Here's how the part is built. I have some questions about the finished solid (model axes, mm). A direction names the side the tool comes from. Give positions to 0.01 mm unless a question says otherwise; leave off trailing zeros. Write each loop counter-clockwise with the first axis right and the second up, starting at its lowest first coordinate (ties: lowest second). Pieces come first, ordered by that corner, then holes. Notation, with made-up numbers: (43, 65.5) - (63, 65.5) arc R32 ccw to (63, 100.5) - close; hole circle Ø2 at (11, 63). An arc over 180 degrees is marked (long way). Use a Markdown table: item, result.
```python
from build123d import *

# Parameters (mm, degrees)
POCKET_DEPTH = 0.75


with BuildPart() as part:
    # Sketch → Revolution (revolve)
    with BuildSketch(Plane.XZ):
        with BuildLine():
            Line((0, 0), (0, 11.75))
            Line((0, 11.75), (2.25, 11.75))
            ThreePointArc((3, 11), (2.78033, 11.53033), (2.25, 11.75))
            Line((3, 11), (3, 10))
            Line((3, 10), (1.5, 10))
            Line((1.5, 10), (1.5, 0))
            Line((1.5, 0), (0, 0))
        make_face()
    revolve(axis=Axis((0, 0, 0), (0, 0, 1)))

    # Sketch001 (on Face5 of Revolution) → Pocket (cut)
    with BuildSketch(Plane(origin=(0, 0, 11.75), x_dir=(-1, 0, 0), z_dir=(0, 0, 1))):
        Polygon((-3.274783, -2.372712), (2.184691, 3.4031), (3.274783, 2.372712), (-2.184691, -3.4031), align=None)
    extrude(amount=-POCKET_DEPTH, mode=Mode.SUBTRACT)


solid = part.part
```
Item 1: If we section it at C-C, the plane z = 8.5: Write out the boundary of the cut face in (x, y).
Values:
| item | result |
|---|---|
| outline | circle Ø3 at (0, 0) |
Item 2: If we section it at B-B, the plane x = 0: Write out the boundary of the cut face in (y, z), plus the area to 3 significant figures.
Values:
| item | result |
|---|---|
| outline | (-3, 10) - (-1.5, 10) - (-1.5, 0) - (1.5, 0) - (1.5, 10) - (3, 10) - (3, 11) arc R0.75 ccw to (2.25, 11.75) - (1.09, 11.75) - (1.09, 11) - (-1.09, 11) - (-1.09, 11.75) - (-2.25, 11.75) arc R0.75 ccw to (-3, 11) - close |
| area | 38.6 mm2 |
Item 3: If we section it at A-A, the plane y = 0: Write out the boundary of the cut face in (x, z), plus the area to 3 significant figures.
Values:
| item | result |
|---|---|
| outline | (-3, 10) - (-1.5, 10) - (-1.5, 0) - (1.5, 0) - (1.5, 10) - (3, 10) - (3, 11) arc R0.75 ccw to (2.25, 11.75) - (1.03, 11.75) - (1.03, 11) - (-1.03, 11) - (-1.03, 11.75) - (-2.25, 11.75) arc R0.75 ccw to (-3, 11) - close |
| area | 38.7 mm2 |
Item 4: I need wall thicknesses on line 1 along Z through (x, y) = (-1.5, -1); line 2 along Z through (x, y) = (-1.75, -0.5); line 3 along Y through (x, z) = (0, 1.25). Which ranges of each line are inside material? Lowest first, please. Write a range as [from, to].
Values:
| item | result |
|---|---|
| line 1 | z = [10, 11] |
| line 2 | z = [10, 11.75] |
| line 3 | y = [-1.5, 1.5] |
Item 5: For faces 1 (the flat face through (0, 0, 11)), 2 (the flat face through (0, 0, 0)), 3 (the flat face through (1.3, -1.3, 10)), which set-ups out of +Z, -Z, +X, -X, +Y, -Y let a thin tool reach every point of the face, with its end or its side?
Values:
| item | result |
|---|---|
| face 1 | +Z |
| face 2 | -Z, +X, -X, +Y, -Y |
| face 3 | -Z |
Item 6: Will these pins go through, and if not, where does the flat tip stop? pin 1 Ø1 at (y, z) = (-0.5, 4.5) entering from +X; pin 2 Ø1.5 at (y, z) = (-0.5, 6.5) entering from -X; pin 3 Ø2 at (x, z) = (-1.5, 1.5) entering from -Y.
Values:
| item | result |
|---|---|
| pin 1 | stops at x = 1.5 |
| pin 2 | stops at x = -1.5 |
| pin 3 | stops at y = -1.41 |
Item 7: Thinking about a two-plate mould opening in X: for faces 4 (the flat face through (-1, 1, 11.75)), 5 (the cylindrical face through (-1.5, 0.07, 4.93)), 6 (the flat face through (0.57, -0.49, 11.38)), which applies, +X half, -X half, draft (parallel to the pull), parting line (faces both ways), or undercut?
Values:
| item | result |
|---|---|
| face 4 | draft |
| face 5 | parting line |
| face 6 | undercut |
